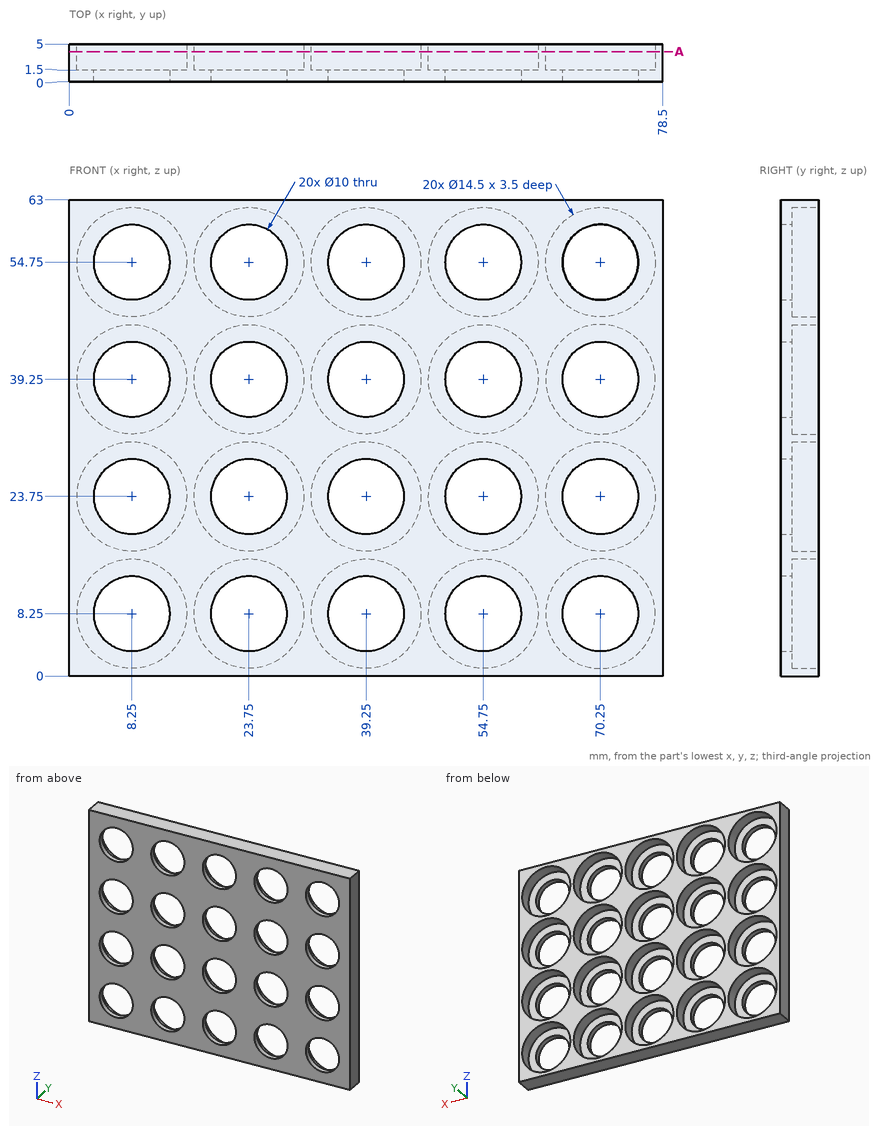
Part print with two shaded views. Sizes in mm from the minimum x, y, z corner. Coordinates: 2 decimals unless noted, no trailing zeros. Answer as a JSON object with one key per item and string values.
Q1. Cut at A-A (y = 4). State how many separate pieces and enclosed holes the cut face has, and give its area (3 significant figures).
Report:
{"separate pieces": "1", "enclosed holes": "20", "area": "1,640 mm2"}
Q2. Flat gauge pins, fed straight in: P1, Ø11.5, axis at x = 25, z = 21.5, coming from the +Y side; P2, Ø8.5, axis at x = 70.25, z = 39.25, coming from the -Y side; P3, Ø4.5, axis at x = 71, z = 11.5, coming from the +Y side. Where does each tip first touch, or does it go through?
Report:
{"P1": "stops at y = 5", "P2": "passes through", "P3": "stops at y = 1.5"}
Q3. Probe probe 1 along Z at (x, y) = (54.75, 2.3); probe 2 along X at (y, z) = (0.5, 8.25); probe 3 along Z at (x, y) = (39.25, 0.65). List the from-to ranges inside material, lowest first.
Report:
{"probe 1": "z = 0 to 1, 15.5 to 16.5, 31 to 32, 46.5 to 47.5, 62 to 63", "probe 2": "x = 0 to 3.25, 13.25 to 18.75, 28.75 to 34.25, 44.25 to 49.75, 59.75 to 65.25, 75.25 to 78.5", "probe 3": "z = 0 to 3.25, 13.25 to 18.75, 28.75 to 34.25, 44.25 to 49.75, 59.75 to 63"}
